Geometry: see drawing. Coordinates: mm, zero at the bounding-box minimum. A direction names the side the tool comes from. Round coordinates to 2 decimals unless told otherwise and drop trailing zeros. Loops run counter-clockwise (first coordinate to the right, second up) from the corner with the lowest first, then second, coordinate; pieces in that order, holes last.
(1) Line query: line 1 (Y direction, x = 2.25, z = 12.5) (1 decimal); line 2 (Z direction, x = 21.5, y = 221) (1 decimal). Output: solid intervals per line, ascending.
(2) Access query for the marked faces 1 and 2. Directions: +Z, -Z, +X, -X, +Y, -Y. A direction counts if a zero-diameter tool reaches every point of the face in a straight line with its end or side. Return the directions, or none.
(3) Cut plane B-B, the plane y = 113. Output: boundary loops of the cut face in (x, z) (1 decimal).
(4) First-contact query: pin 1 Ø11 at (y, z) = (170, 13) entering from +X (1 decimal). Flat tip, straight axial feed; report the tip coordinate or a pass-through.
(5) Cut plane C-C, the plane x = 21.5. Output: boundary loops of the cut face in (y, z) (1 decimal).
(6) Cut plane A-A, the plane z = 15.25. Output: boundary loops of the cut face in (x, y) (1 decimal).
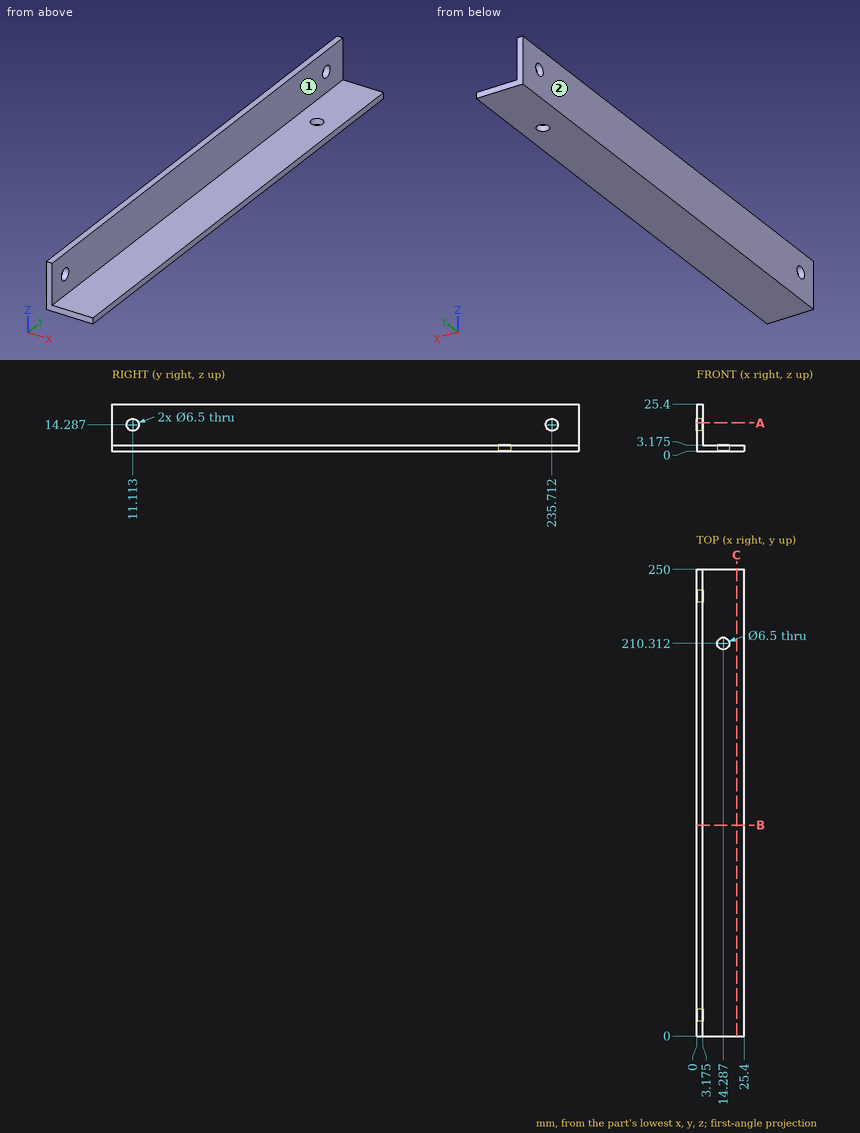
Reported:
1. line 1: y = 0 to 8.4, 13.8 to 233, 238.4 to 250
1. line 2: z = 0 to 3.2
2. face 1: +Z, +X, +Y, -Y
2. face 2: +Z, -Z, -X, +Y, -Y
3. outline: (0, 0) - (25.4, 0) - (25.4, 3.2) - (3.2, 3.2) - (3.2, 25.4) - (0, 25.4) - close
4. pin 1: stops at x = 3.2
5. outline: (0, 0) - (250, 0) - (250, 3.2) - (0, 3.2) - close
6. outline: (0, 0) - (3.2, 0) - (3.2, 8) - (0, 8) - close; (0, 14.2) - (3.2, 14.2) - (3.2, 232.6) - (0, 232.6) - close; (0, 238.8) - (3.2, 238.8) - (3.2, 250) - (0, 250) - close
